The figure shows three views and two pictorial views of one solid part (mm, origin at its lowest corner). Answer the questions. A direction names the side the tool comes from. Give positions to 0.01 mm unless a question says otherwise; leave off trailing zeros. Order: outer loops, then holes, each group sorted by start corner. A loop starts at its lowest first (then second) coordinate and runs counter-clockwise, first axis right, second up. Notation, with made-up numbers: (77.25, -23) - (112.25, -23) arc R20 ccw to (112.25, 13) - close; hole circle Ø3 at (41.25, 44.5). An arc over 180 degrees is marked (long way). Write item = value, one per line.
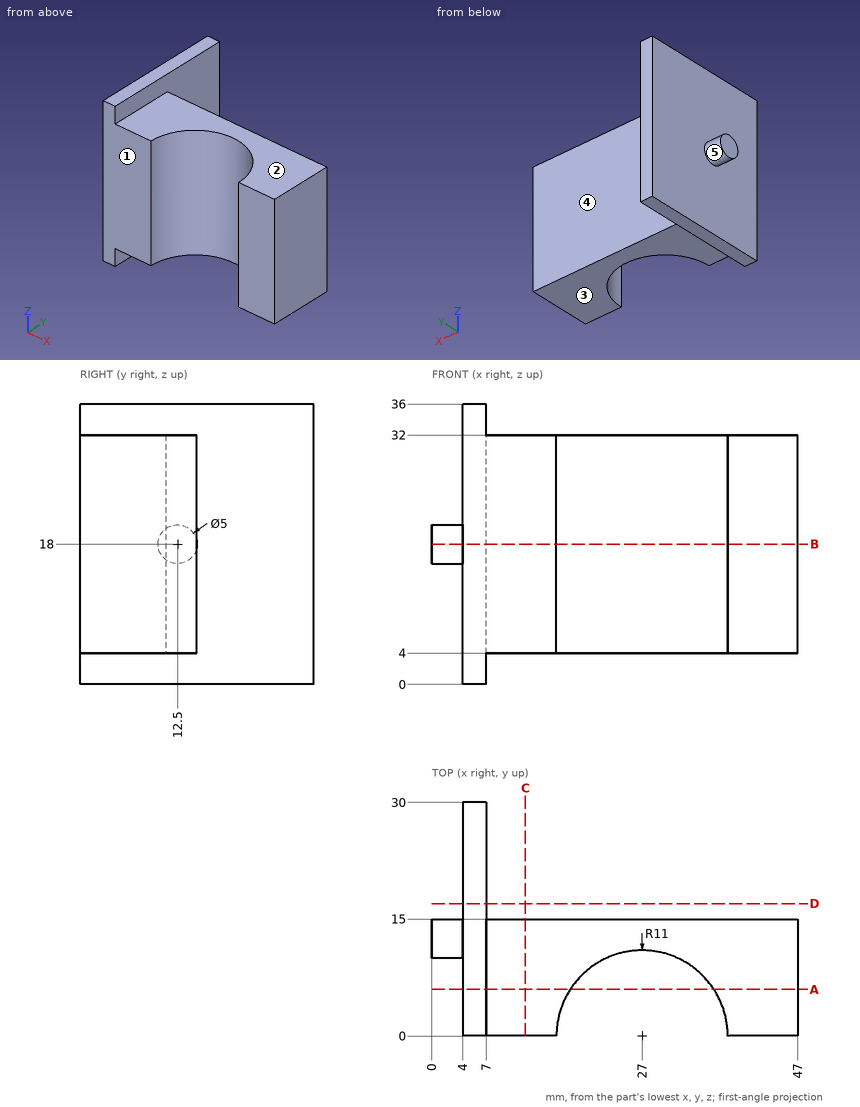
1. Flat-ended cylindrical pins translate along their axes: pin 1 (4 mm diameter, centred on x = 29.5, y = 7, fed in from +Z); pin 2 (16.5 mm diameter, centred on x = 20.5, y = 11, fed in from -Z); pin 3 (1 mm diameter, centred on x = 35, z = 24.5, fed in from +Y); pin 4 (1.5 mm diameter, centred on y = 17, z = 16, fed in from -X). Find the tip coordinate at first contact, or state that the pin passes through.
Recorded:
pin_1 = through
pin_2 = 4
pin_3 = 15
pin_4 = 4
2. Straight lines are drawn through the part: L1, parallel to Y at x = 43.5, z = 22; L2, parallel to X at y = 23.5, z = 23.5; L3, parallel to Z at x = 11.5, y = 8.5. For each, find the intervals that lie inside material, in ascending order. Write a range as [from, to].
Recorded:
L1 = [0, 15]
L2 = [4, 7]
L3 = [4, 32]
3. For the marked faces 1, 2, 3, 4 and 5, determine the directions among +Z, -Z, +X, -X, +Y, -Y from which every point of the face is accessible in a straight line to the end or side of a thin tool.
Recorded:
face_1 = +Z, -Z, +X, -X, -Y
face_2 = +Z, +X, +Y, -Y
face_3 = -Z, +X, +Y, -Y
face_4 = +Z, -Z, +X, +Y
face_5 = -X
4. Section A-A (y = 6) is taken. Determine the outline of the cut face in (x, z), and give its area (3 significant figures).
Recorded:
outline = (4, 0) - (7, 0) - (7, 4) - (17.78, 4) - (17.78, 32) - (7, 32) - (7, 36) - (4, 36) - close; (36.22, 4) - (47, 4) - (47, 32) - (36.22, 32) - close
area = 712 mm^2
5. Section C-C (x = 12) is taken. Determine the outline of the cut face in (y, z), and give its area (3 significant figures).
Recorded:
outline = (0, 4) - (15, 4) - (15, 32) - (0, 32) - close
area = 420 mm^2
6. Section D-D (y = 17) is taken. Determine the outline of the cut face in (x, z).
Recorded:
outline = (4, 0) - (7, 0) - (7, 36) - (4, 36) - close
7. Section B-B (z = 18) is taken. Determine the outline of the cut face in (x, y), and give its area (3 significant figures).
Recorded:
outline = (0, 10) - (4, 10) - (4, 0) - (16, 0) arc R11 cw to (38, 0) - (47, 0) - (47, 15) - (7, 15) - (7, 30) - (4, 30) - (4, 15) - (0, 15) - close
area = 520 mm^2
